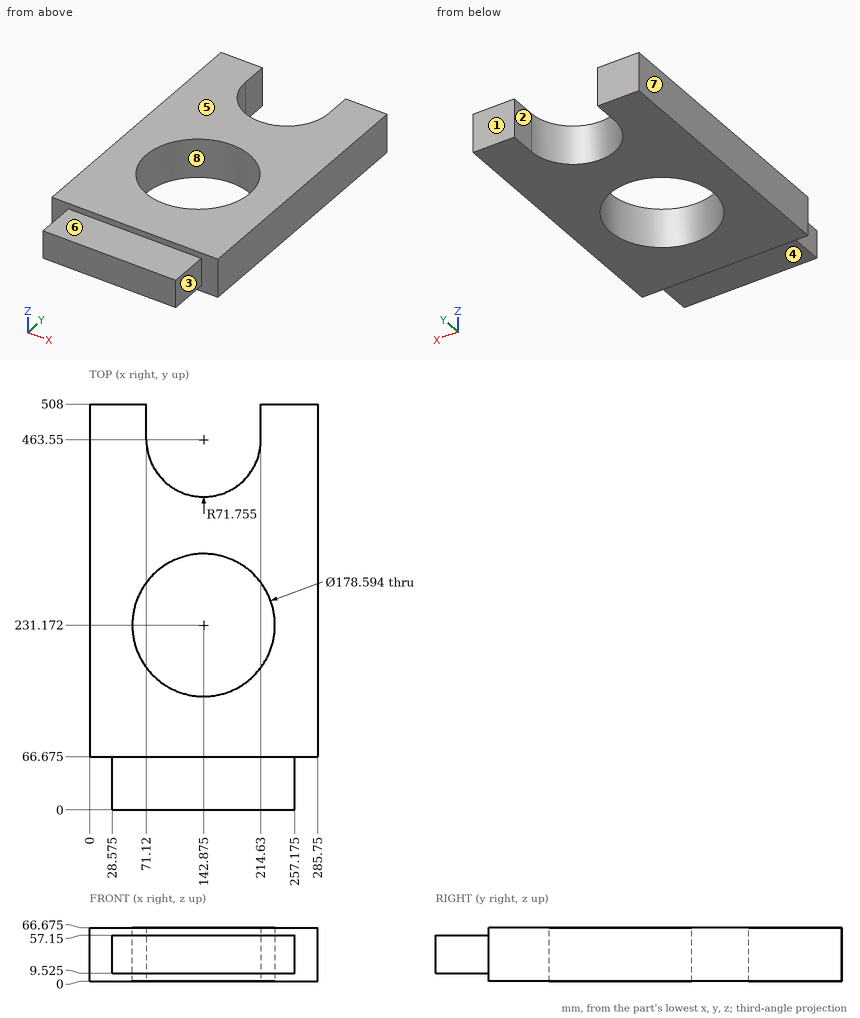
Input: dimensioned drawing with shaded views. Units: mm. Origin: part minimum x, y, z. A direction names the side the tool comes from. Coordinates: 2 decimals unless noted, no trailing zeros. One line per item, written item: value. Start each with the question number.
Q1. Set-up query: the marked faces 1, 2, 3, 4 and 5. Return all of +Z, -Z, +X, -X, +Y, -Y with unobstructed straight access to the full face (end or side cutting, diameter ignored); none if empty.
Q2. Mould query, pull axis X, two halves, no side actions, for the marked faces 6, 7 and 8. Classes: pulls with the +X half, pulls with the -X half, needs draft (parallel to the pull), parting line crosses it, or undercut.
Q3. Line query: line 1 along X through (y, z) = (466.5, 6.5); line 2 along Y through (x, z) = (63.5, 50) (1 decimal); line 3 along X through (y, z) = (239, 28). Output: solid intervals per line, ascending.
Q4. Contact query for flat-ended pins moving along their axis: P1, Ø20, axis at x = 126.5, y = 37.5, coming from the -Z side (3 decimals); P2, Ø14.5, axis at y = 27.5, z = 23, coming from the +X side (3 decimals). Output: stop coordinate, or through.
Results:
1. face 1: +Z, -Z, +X, -X, +Y
1. face 2: +Z, -Z, +Y
1. face 3: +Z, -Z, +X, -Y
1. face 4: -Z, +X, -X, -Y
1. face 5: +Z, +X, -X, +Y, -Y
2. face 6: needs draft
2. face 7: pulls with the -X half
2. face 8: undercut
3. line 1: 0 to 71.12, 214.63 to 285.75
3. line 2: 0 to 190.3, 272.1 to 508
3. line 3: 0 to 53.92, 231.83 to 285.75
4. P1: z = 9.525
4. P2: x = 257.175
